Read the model definition and answer for the solid it produces. Units are mm, in the model's axes. A direction names the side the tool comes from. Coordinates: 2 decimals unless noted, no trailing zeros. Order: outer loops, then holes, each group sorted by start corner. A loop starts at its lowest first (then second) coordinate and runs counter-clockwise, first axis right, second up. Notation, with made-up numbers: M -34.75,-15.75 L 19.25,-15.75 A6 cw 19.25,-7.75 Z; hole C 16,12.5 d7. An arc over 180 degrees is marked long. Put each result on its own line as item: value.
from build123d import *

# Parameters (mm, degrees)
SKETCH1_W           = 19.1008
SKETCH1_H           = 6.4008
BOSS_EXTRUDE1_DEPTH = 1.905
SKETCH2_W           = 13.081
SKETCH2_H           = 6.4008
BOSS_EXTRUDE2_DEPTH = 1.143
CUT_EXTRUDE1_REACH  = 5.048
SKETCH3_R           = 0.762
CUT_EXTRUDE2_REACH  = 5.048
SKETCH4_R           = 1.5875


with BuildPart() as part:
    # Sketch1 → Boss-Extrude1 (new body)
    with BuildSketch(Plane(origin=(0, 0, 0), x_dir=(1, 0, 0), z_dir=(0, 1, 0))):
        Rectangle(SKETCH1_W, SKETCH1_H)
    extrude(amount=BOSS_EXTRUDE1_DEPTH)

    # Sketch2 → Boss-Extrude2 (add)
    with BuildSketch(Plane(origin=(0, 0, 0), x_dir=(-1, 0, 0), z_dir=(0, -1, 0))):
        with Locations((-3.0099, 0)):
            Rectangle(SKETCH2_W, SKETCH2_H)
    extrude(amount=BOSS_EXTRUDE2_DEPTH)

    # Sketch3 → Cut-Extrude1 (cut, up to next)
    with BuildSketch(Plane(origin=(0, 1.905, 0), x_dir=(1, 0, 0), z_dir=(0, 1, 0)), mode=Mode.PRIVATE) as cut_extrude1_sk1:
        with Locations((-8.2804, 0)):
            Circle(SKETCH3_R)
    cut_extrude1_tool1 = extrude(cut_extrude1_sk1.sketch, amount=-CUT_EXTRUDE1_REACH, mode=Mode.PRIVATE) & part.part
    add(cut_extrude1_tool1.solids().sort_by_distance((-8.2804, 1.905, 0))[0], mode=Mode.SUBTRACT)

    # Sketch4 → Cut-Extrude2 (cut, up to next)
    with BuildSketch(Plane(origin=(0, 1.905, 0), x_dir=(1, 0, 0), z_dir=(0, 1, 0)), mode=Mode.PRIVATE) as cut_extrude2_sk1:
        with Locations((3.81, 0)):
            Circle(SKETCH4_R)
    cut_extrude2_tool1 = extrude(cut_extrude2_sk1.sketch, amount=-CUT_EXTRUDE2_REACH, mode=Mode.PRIVATE) & part.part
    add(cut_extrude2_tool1.solids().sort_by_distance((3.81, 1.905, 0))[0], mode=Mode.SUBTRACT)


solid = part.part
Q1. Find section B-B on x = 3.81. Write down the section's boundary in (y, z) (1 decimal), plus the area to 3 significant figures.
Answers below:
outline: M -1.1,-3.2 L 1.9,-3.2 L 1.9,-1.6 L -1.1,-1.6 Z; M -1.1,1.6 L 1.9,1.6 L 1.9,3.2 L -1.1,3.2 Z
area: 9.83 mm^2
Q2. Given pin 1 (0.9 mm diameter, centred on y = -1, z = 0.5, fed in from -X); pin 2 (1.2 mm diameter, centred on x = -8.28, z = 0, fed in from +Y), each flat-ended and moving along its own axis, determine where each tip first touches the part or whether it passes through.
Answers below:
pin 1: stops at x = -3.53
pin 2: passes through
Q3. A tool of negligible diameter and unlimited length cuts with its end or side. For faces 1 (the face through (-9.55, 1, 0)), 2 (the face through (-7, 0, 0)), from which of +Z, -Z, +X, -X, +Y, -Y can it reach the whole face along a straight path? Write none if from no direction.
Answers below:
face 1: +Z, -Z, -X, +Y, -Y
face 2: +Z, -Z, -X, -Y
Q4. Find section C-C on y = -0.6. Write down the section's boundary in (x, z) (1 decimal).
Answers below:
outline: M -3.5,-3.2 L 9.6,-3.2 L 9.6,3.2 L -3.5,3.2 Z; hole C 3.8,0 d3.2
Q5. Consider line 1 along X through (y, z) = (1.2, 0); line 2 along Z through (x, y) = (3.81, 1.1); line 3 along X through (y, z) = (0.4, -0.5). Determine where each line is inside the solid, lowest interval first.
Answers below:
line 1: x = -9.55 to -9.04, -7.52 to 2.22, 5.4 to 9.55
line 2: z = -3.2 to -1.59, 1.59 to 3.2
line 3: x = -9.55 to -8.86, -7.71 to 2.3, 5.32 to 9.55
Q6. Find section D-D on y = 1.2. Write down the section's boundary in (x, z) (1 decimal).
Answers below:
outline: M -9.6,-3.2 L 9.6,-3.2 L 9.6,3.2 L -9.6,3.2 Z; hole C -8.3,0 d1.5; hole C 3.8,0 d3.2
Q7. For a pull along Z with two mould halves and no side action, classify faces 3 (the face through (0, 0, 3.2)), 4 (the face through (-3.531, -0.6, 0)), 5 (the face through (-9.04, 0.97, -0.03)) as +Z half, -Z half, draft (parallel to the pull), parting line (faces both ways), or undercut.
Answers below:
face 3: +Z half
face 4: draft
face 5: undercut
Q8. Find section A-A on z = 0. Write down the section's boundary in (x, y) (1 decimal).
Answers below:
outline: M -9.6,0 L -9,0 L -9,1.9 L -9.6,1.9 Z; M -7.5,0 L -3.5,0 L -3.5,-1.1 L 2.2,-1.1 L 2.2,1.9 L -7.5,1.9 Z; M 5.4,-1.1 L 9.6,-1.1 L 9.6,1.9 L 5.4,1.9 Z
